The model under review builds one solid part; all positions refer to its coordinate system, in mm. Face numbers are marked on the shaded views. Round coordinates to 2 decimals unless told otherwise and drop trailing zeros. Order: outer loops, then holes, each group sorted by start corner. A loop starts at its lowest first (then second) coordinate and runs counter-clockwise, first axis right, second up.
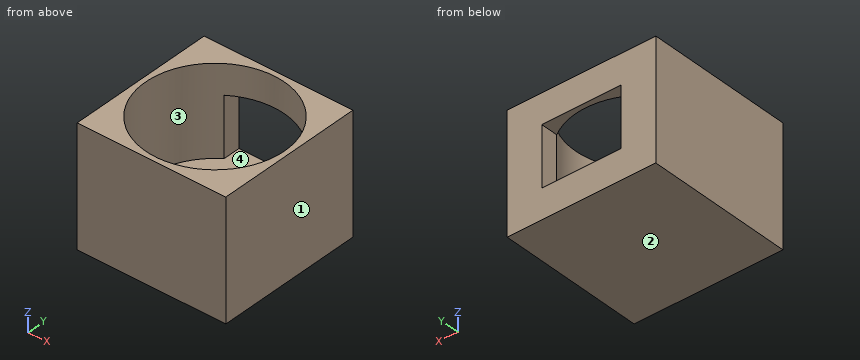
```python
from build123d import *

# Parameters (mm, degrees)
CROQUIS1_W              = 15
CROQUIS1_H              = 15
SALIENTE_EXTRUIR1_DEPTH = 12
CROQUIS2_W              = 8
CROQUIS2_H              = 6
CORTAR_EXTRUIR1_DEPTH   = 10
CROQUIS3_R              = 7
CORTAR_EXTRUIR2_DEPTH   = 9


with BuildPart() as part:
    # Croquis1 → Saliente-Extruir1 (new body)
    with BuildSketch(Plane.XY):
        Rectangle(CROQUIS1_W, CROQUIS1_H)
    extrude(amount=SALIENTE_EXTRUIR1_DEPTH)

    # Croquis2 → Cortar-Extruir1 (cut)
    with BuildSketch(Plane(origin=(0, 7.5, 0), x_dir=(1, 0, 0), z_dir=(0, 1, 0))):
        with Locations((0, -6)):
            Rectangle(CROQUIS2_W, CROQUIS2_H)
    extrude(amount=-CORTAR_EXTRUIR1_DEPTH, mode=Mode.SUBTRACT)

    # Croquis3 → Cortar-Extruir2 (cut)
    with BuildSketch(Plane.XY.offset(12)):
        Circle(CROQUIS3_R)
    extrude(amount=-CORTAR_EXTRUIR2_DEPTH, mode=Mode.SUBTRACT)


solid = part.part
```
(1) Insertion check: pin 1 (4 mm diameter, centred on x = -1, y = 0.5, fed in from +Z). The pin has a flat end and moves straight along its axis. Give the tip position at first contact, or say it passes through.
Data:
pin 1: stops at z = 3
(2) Consider section B-B (z = 7). Write out the cut boundary in (x, y).
Data:
outline: (-7.5, -7.5) - (7.5, -7.5) - (7.5, 7.5) - (4, 7.5) - (4, 5.74) arc R7 cw (long way) to (-4, 5.74) - (-4, 7.5) - (-7.5, 7.5) - close
(3) Consider section C-C (y = 0). Write out the cut boundary in (x, z), and give its area (3 significant figures).
Data:
outline: (-7.5, 0) - (7.5, 0) - (7.5, 12) - (7, 12) - (7, 3) - (-7, 3) - (-7, 12) - (-7.5, 12) - close
area: 54.0 mm2
(4) Consider section D-D (x = 1.75). Write out the cut boundary in (y, z), and give its area (3 significant figures).
Data:
outline: (-7.5, 0) - (7.5, 0) - (7.5, 3) - (-6.78, 3) - (-6.78, 12) - (-7.5, 12) - close; (6.78, 9) - (7.5, 9) - (7.5, 12) - (6.78, 12) - close
area: 53.7 mm2
(5) Draft analysis for pull direction X (two halves, no side actions). For the marked faces 1, 2, 3 and 4, state which applies: pulls with the +X half, pulls with the -X half, needs draft (parallel to the pull), parting line crosses it, or undercut.
Data:
face 1: pulls with the +X half
face 2: needs draft
face 3: undercut
face 4: undercut
(6) Consider section A-A (x = 0). Write out the cut boundary in (y, z).
Data:
outline: (-7.5, 0) - (7.5, 0) - (7.5, 3) - (-7, 3) - (-7, 12) - (-7.5, 12) - close; (7, 9) - (7.5, 9) - (7.5, 12) - (7, 12) - close
(7) To check wall thickness, follow probe 1 along X at (y, z) = (0, 9); probe 2 along X at (y, z) = (6.5, 4.75); probe 3 along Z at (x, y) = (3.5, 6.25). State the ranges of each line that lie inside material, in increasing order.
Data:
probe 1: x = -7.5 to -7, 7 to 7.5
probe 2: x = -7.5 to -4, 4 to 7.5
probe 3: z = 0 to 3, 9 to 12
